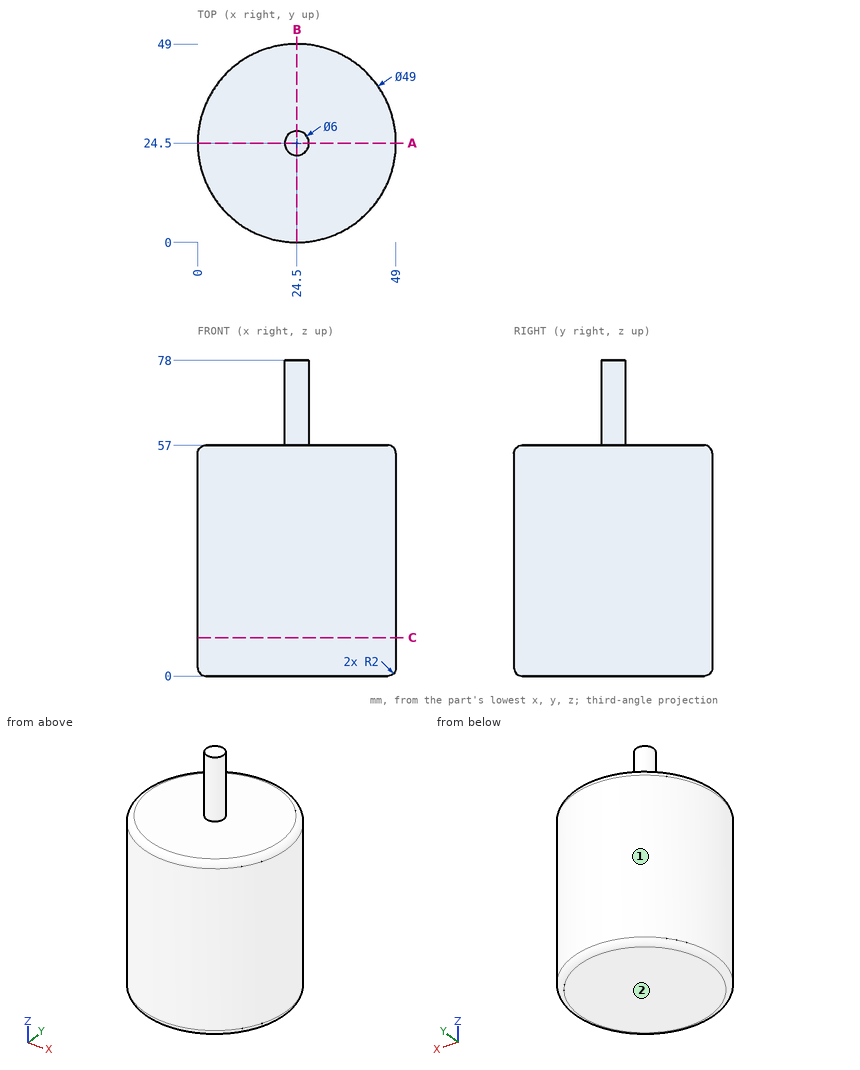
Geometry check sheet. Reference: drawing and pictorial views, mm from the part's lowest x, y, z. Round coordinates to 2 decimals unless told otherwise and drop trailing zeros. Order: outer loops, then holes, each group sorted by start corner. A loop starts at its lowest first (then second) coordinate and runs counter-clockwise, first axis right, second up. Notation, with made-up numbers: (-26, -2.75) - (32, -2.75) arc R24 cw to (32, 14.25) - close; hole circle Ø2 at (-34, 49). An arc over 180 degrees is marked (long way). Write item = value, one per line.
Q1. Thickness scan on line 1 along Z through (x, y) = (32, 21); line 2 along X through (y, z) = (33, 48); line 3 along X through (y, z) = (42.5, 29). Record the ranges inside material, lowest first.
Computed:
line_1 = 0 to 57
line_2 = 1.52 to 47.48
line_3 = 7.88 to 41.12
Q2. Section check C-C (z = 9.5). Record the boundary of the cut face in (x, y).
Computed:
outline = circle Ø49 at (24.5, 24.5)
Q3. Section check A-A (y = 24.5). Record the boundary of the cut face in (x, z).
Computed:
outline = (0, 2) arc R2 ccw to (2, 0) - (47, 0) arc R2 ccw to (49, 2) - (49, 55) arc R2 ccw to (47, 57) - (27.5, 57) - (27.5, 78) - (21.5, 78) - (21.5, 57) - (2, 57) arc R2 ccw to (0, 55) - close
Q4. Go/stop test with flat-tipped pins: pin 1 (5 mm diameter, centred on y = 40, z = 33, fed in from -X); pin 2 (8 mm diameter, centred on y = 29, z = 30.5, fed in from +X). Record where each tip stops, or that it passes through.
Computed:
pin_1 = 3.73
pin_2 = 48.99
Q5. Draft check along X on the marked faces 1 and 2. Enter one of: pulls with the +X half, pulls with the -X half, needs draft (parallel to the pull), parting line crosses it, or undercut.
Computed:
face_1 = parting line crosses it
face_2 = needs draft
